from build123d import *

# Parameters (mm, degrees)
SKETCH1_W                        = 44.45
SKETCH1_H                        = 44.45
SKETCH1_W_2                      = 38.1
SKETCH1_H_2                      = 38.1
BOSS_EXTRUDE1_DEPTH              = 844.55
F_17_64_0_26563_DIAMETER_HOLE1_D = 6.747002
SKETCH6_R                        = 3.3734375
CUT_EXTRUDE1_DEPTH               = 847.010907509


with BuildPart() as part:
    # Sketch1 → Boss-Extrude1 (new body)
    with BuildSketch(Plane(origin=(0, 0, 0), x_dir=(1, 0, 0), z_dir=(0, 1, 0))):
        Rectangle(SKETCH1_W, SKETCH1_H)
        Rectangle(SKETCH1_W_2, SKETCH1_H_2, mode=Mode.SUBTRACT)
    extrude(amount=BOSS_EXTRUDE1_DEPTH)

    # 17/64 (0.26563) Diameter Hole1 (through all)
    with Locations(Plane.XY.offset(22.225)):
        with Locations((0, 768.35), (0, 76.2)):
            Hole(F_17_64_0_26563_DIAMETER_HOLE1_D / 2)

    # Sketch6 → Cut-Extrude1 (cut, through all)
    with BuildSketch(Plane(origin=(22.225, 0, 0), x_dir=(0, 0, -1), z_dir=(1, 0, 0))):
        with Locations((0, 136.525)):
            Circle(SKETCH6_R)
        with Locations((0, 708.025)):
            Circle(SKETCH6_R)
    extrude(amount=-CUT_EXTRUDE1_DEPTH, mode=Mode.SUBTRACT)


solid = part.part
The model under review builds one solid part; all positions refer to its coordinate system, in mm. A direction names the side the tool comes from. Give positions to 0.01 mm unless a question says otherwise; leave off trailing zeros. Write each loop counter-clockwise with the first axis right and the second up, starting at its lowest first coordinate (ties: lowest second). Pieces come first, ordered by that corner, then holes.
1. Draft analysis for pull direction Z (two halves, no side actions). For faces 1 (the flat face through (-19.05, 416, 0)), 2 (the flat face through (0, 416, -22.225)), 3 (the flat face through (0, 416, 22.225)), 4 (the flat face through (19.4, 0, -0.3)), state which applies: +Z half, -Z half, draft (parallel to the pull), parting line (faces both ways), or undercut.
2. Add section B-B, the plane y = 638.5. Write out the cut boundary in (x, z) (3 decimals), plus the area to 3 significant figures.
3. Wall thickness on L1, parallel to Y at x = -19.95, z = 0; L2, parallel to Z at x = 12.5, y = 721 (3 decimals): over which ranges is each line inside the solid? List them lowest first.
4. Tool access review of faces 5 (the flat face through (19.05, 416, 0)), 6 (the flat face through (19.4, 844.55, -0.3)): name each direction out of +Z, -Z, +X, -X, +Y, -Y from which nothing blocks a thin tool from reaching the whole face with its end or side.
5. Add section A-A, the plane x = -10.5. Write out the cut boundary in (y, z) (3 decimals), plus the area to 3 significant figures.
6. For P1, Ø6, axis at x = 0, y = 76.2, coming from the +Z side, flat-tipped, find the tip position at first contact; note if it passes through.
Worked answers:
1. face 1: undercut
1. face 2: -Z half
1. face 3: +Z half
1. face 4: draft
2. outline: (-22.225, -22.225) - (22.225, -22.225) - (22.225, 22.225) - (-22.225, 22.225) - close; hole (-19.05, -19.05) - (19.05, -19.05) - (19.05, 19.05) - (-19.05, 19.05) - close
2. area: 524 mm2
3. L1: y = 0 to 133.15, 139.9 to 704.65, 711.4 to 844.55
3. L2: z = -22.225 to -19.05, 19.05 to 22.225
4. face 5: +Y, -Y
4. face 6: +Z, -Z, +X, -X, +Y
5. outline: (0, -22.225) - (844.55, -22.225) - (844.55, -19.05) - (0, -19.05) - close; (0, 19.05) - (844.55, 19.05) - (844.55, 22.225) - (0, 22.225) - close
5. area: 5,360 mm2
6. P1: passes through
